Here's the drawing with two shaded views (mm, measured from the low corner). I have some questions. Coordinates: 2 decimals unless noted, no trailing zeros. Write each loop counter-clockwise with the first axis right and the second up, starting at its lowest first coordinate (ties: lowest second). Pieces come first, ordered by that corner, then holes.
Item 1: If we section it at A-A (x = 8): Please give me the cut outline in (y, z).
Item 2: If we section it at B-B (y = 23): Please give me the cut outline in (x, z), then the cut area to 3 significant figures.
Item 3: I'm going to push a flat-ended pin straight in: pin 1 Ø1.5 at (x, z) = (26.5, 5.5) entering from -Y. Where does the tip first touch, or does it pass through?
Item 4: If I drill on line 1 (Y direction, x = 30, z = 6); line 2 (X direction, y = 8.5, z = 4.75); line 3 (Y direction, x = 7.5, z = 8), over which ranges is the centre line in solid material (lowest first)?
Item 5: If we section it at D-D (z = 8): Please give me the cut outline in (x, y), then the cut area to 3 significant figures.
Item 6: If we section it at C-C (y = 8): Please give me the cut outline in (x, z).
Item 7: We'd pull the mould along X, two halves only. Please class the marked faces 1, 2 and 3: +X half, -X half, draft (parallel to the pull), parting line (faces both ways), or undercut.
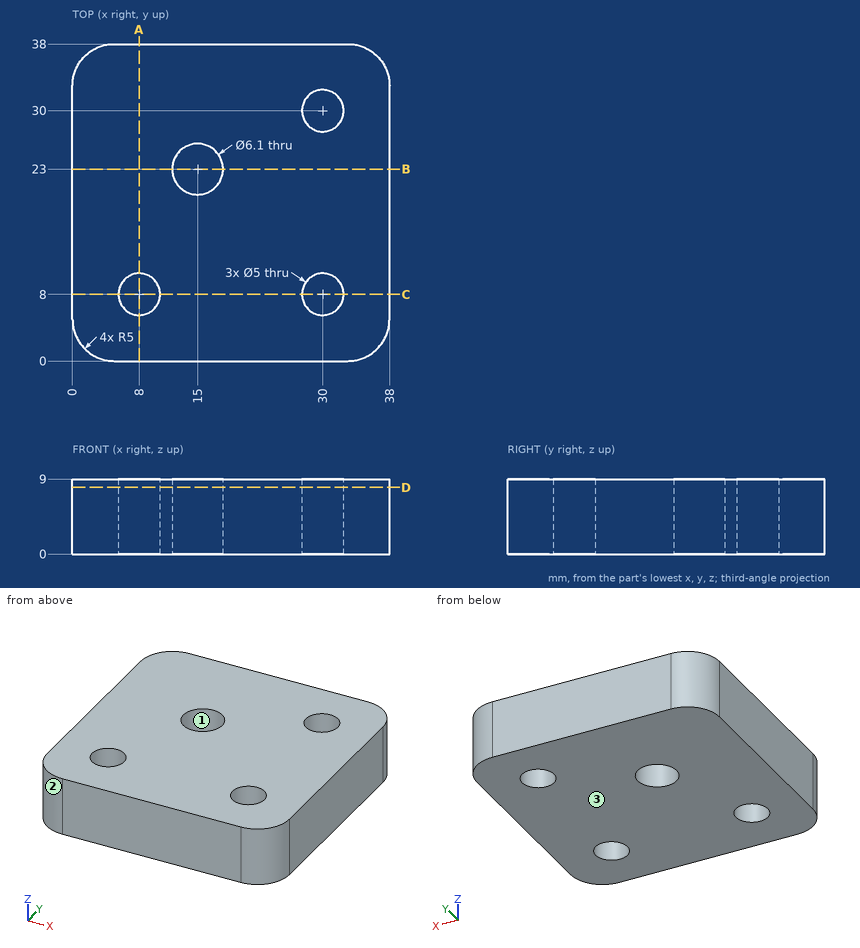
Answer list:
1. outline: (0, 0) - (5.5, 0) - (5.5, 9) - (0, 9) - close; (10.5, 0) - (38, 0) - (38, 9) - (10.5, 9) - close
2. outline: (0, 0) - (11.95, 0) - (11.95, 9) - (0, 9) - close; (18.05, 0) - (38, 0) - (38, 9) - (18.05, 9) - close
2. area: 287 mm2
3. pin 1: stops at y = 0
4. line 1: y = 0 to 5.5, 10.5 to 27.5, 32.5 to 38
4. line 2: x = 0 to 5.55, 10.45 to 27.55, 32.45 to 38
4. line 3: y = 0 to 5.55, 10.45 to 38
5. outline: (0, 5) arc R5 ccw to (5, 0) - (33, 0) arc R5 ccw to (38, 5) - (38, 33) arc R5 ccw to (33, 38) - (5, 38) arc R5 ccw to (0, 33) - close; hole circle Ø5 at (8, 8); hole circle Ø6.1 at (15, 23); hole circle Ø5 at (30, 8); hole circle Ø5 at (30, 30)
5. area: 1,330 mm2
6. outline: (0, 0) - (5.5, 0) - (5.5, 9) - (0, 9) - close; (10.5, 0) - (27.5, 0) - (27.5, 9) - (10.5, 9) - close; (32.5, 0) - (38, 0) - (38, 9) - (32.5, 9) - close
7. face 1: undercut
7. face 2: -X half
7. face 3: draft
